from build123d import *

# Parameters (mm, degrees)
SKETCH_1_R          = 2.05
EXTRUDE_1_DEPTH     = 20
FILLET_1_R          = 12
FILLET_2_R          = 8
FILLET_3_R          = 1
FILLET_4_R          = 25
SKETCH_6_R          = 4
CUT_EXTRUDE_5_DEPTH = 3
SKETCH_7_R          = 1.25
CUT_EXTRUDE1_DEPTH  = 10
CUT_EXTRUDE2_START  = -3
SKETCH1_R           = 4
CUT_EXTRUDE2_DEPTH  = 3


with BuildPart() as part:
    # 草图1 → 凸台-拉伸1 (new body)
    with BuildSketch(Plane.XY):
        with BuildLine():
            Line((13.750969278, -0.819876155), (13.750969278, -0.183047918))
            ThreePointArc((13.750969278, -0.183047918), (0.091525986, 13.751882984), (-13.752187557, 0))
            ThreePointArc((-13.752187557, 0), (-24.470803545, -4.924054358), (-35.721657685, -8.467120986))
            ThreePointArc((-35.721657685, -8.467120986), (-46.713142569, -1.298230159), (-54.919247866, -11.538619386))
            Line((-54.919247866, -11.538619386), (-55, -11.852756493))
            Line((-55, -11.852756493), (-55, -22.177115611))
            Line((-55, -22.177115611), (-45.17004572, -22.177115611))
            ThreePointArc((-45.17004572, -22.177115611), (2.155746263, -16.550210115), (49.481538246, -22.177115611))
            Line((49.481538246, -22.177115611), (60, -22.177115611))
            Line((60, -22.177115611), (60, -15.54238751))
            ThreePointArc((60, -15.54238751), (36.185940998, -10.347251745), (13.750969278, -0.819876155))
        make_face()
        with Locations((-45.17004572, -10.942949795)):
            Circle(SKETCH_1_R, mode=Mode.SUBTRACT)
        with BuildLine():
            Line((-7.5, -2.5), (-7.5, 2.5))
            Line((-7.5, 2.5), (-4.330127019, 2.5))
            ThreePointArc((-4.330127019, 2.5), (0, 5), (4.330127019, 2.5))
            Line((4.330127019, 2.5), (7.5, 2.5))
            Line((7.5, 2.5), (7.5, -2.5))
            Line((7.5, -2.5), (4.330127019, -2.5))
            ThreePointArc((4.330127019, -2.5), (0, -5), (-4.330127019, -2.5))
            Line((-4.330127019, -2.5), (-7.5, -2.5))
        make_face(mode=Mode.SUBTRACT)
    extrude(amount=EXTRUDE_1_DEPTH)

    # 圆角1
    fillet_1_edges = [part.edges().sort_by_distance(p)[0] for p in [
        (-13.752187557, 0, 10),
    ]]
    fillet(fillet_1_edges, radius=FILLET_1_R)

    # 圆角2
    fillet_2_edges = [part.edges().sort_by_distance(p)[0] for p in [
        (-35.721657685, -8.467120986, 10),
    ]]
    fillet(fillet_2_edges, radius=FILLET_2_R)

    # 圆角3
    fillet_3_edges = [part.edges().sort_by_distance(p)[0] for p in [
        (60, -15.54238751, 10),
        (60, -22.177115611, 10),
        (-55, -22.177115611, 10),
    ]]
    fillet(fillet_3_edges, radius=FILLET_3_R)

    # 圆角4
    fillet_4_edges = [part.edges().sort_by_distance(p)[0] for p in [
        (13.750969278, -0.819876155, 10),
    ]]
    fillet(fillet_4_edges, radius=FILLET_4_R)

    # 草图6 → 切除-拉伸5 (cut)
    with BuildSketch(Plane(origin=(0, 0, 0), x_dir=(-1, 0, 0), z_dir=(0, 0, -1))):
        with Locations((45.17004572, -10.942949795)):
            Circle(SKETCH_6_R)
    extrude(amount=-CUT_EXTRUDE_5_DEPTH, mode=Mode.SUBTRACT)

    # 草图7 → Cut-Extrude1 (cut)
    with BuildSketch(Plane.XY):
        with Locations((-49.334528207, -19.024990649)):
            Circle(SKETCH_7_R)
        with Locations((54.787690727, -19.024990649)):
            Circle(SKETCH_7_R)
        with Locations((34.734293207, -16.420229149)):
            Circle(SKETCH_7_R)
        with Locations((-28.075836585, -16.420229149)):
            Circle(SKETCH_7_R)
    extrude(amount=CUT_EXTRUDE1_DEPTH, mode=Mode.SUBTRACT)

    # Sketch1 → Cut-Extrude2 (cut)
    with BuildSketch(Plane.XY.offset(20).offset(CUT_EXTRUDE2_START)):
        with Locations(Location((-45.17004572, -10.942949795, 0), (0, 0, 180))):
            Circle(SKETCH1_R)
    extrude(amount=CUT_EXTRUDE2_DEPTH, mode=Mode.SUBTRACT)


solid = part.part
The model under review builds one solid part; all positions refer to its coordinate system, in mm. A direction names the side the tool comes from. Give positions to 0.01 mm unless a question says otherwise; leave off trailing zeros. Loops run counter-clockwise (first coordinate to the right, second up) from the corner with the lowest first, then second, coordinate; pieces in that order, holes last. Notation, with made-up numbers: (62, 34) -> (102, 34) arc R18 ccw to (102, 52) -> close; hole circle Ø5 at (88.5, 31). An arc over 180 degrees is marked (long way). Write each question's results on one line, items separated by ' | '.
1) Draft analysis for pull direction X (two halves, no side actions). For faces 5 (the face through (2, -8, 0)), 6 (the face through (-41.174, -11.119, 18.479)), 7 (the face through (42.14, -12.09, 9.86)), state which applies: pulls with the +X half, pulls with the -X half, needs draft (parallel to the pull), parting line crosses it, or undercut.
Conclusion:
face 5: needs draft | face 6: undercut | face 7: pulls with the +X half
2) Take a section at B-B, the plane z = 7.5. Count the separate pieces of the cut face and the enclosed holes in it, plus the area to 3 significant figures.
Conclusion:
separate pieces: 1 | enclosed holes: 6 | area: 1,760 mm^2
3) Insertion check: pin 1 Ø4 at (y, z) = (-1, 15) entering from -X; pin 2 Ø1 at (x, z) = (-5.5, 5.5) entering from -Y; pin 3 Ø4 at (y, z) = (0.5, 6.5) entering from +X. Each pin has a flat end and moves straight along its axis. Give the tip position at first contact, or say it passes through.
Conclusion:
pin 1: stops at x = -50.85 | pin 2: stops at y = -16.72 | pin 3: stops at x = 17.84
4) Take a section at C-C, the plane y = 7.5. Give the boundary of the cut face in (x, z), plus the area to 3 significant figures.
Conclusion:
outline: (-11.53, 0) -> (11.53, 0) -> (11.53, 20) -> (-11.53, 20) -> close | area: 461 mm^2
5) For line 1 along X through (y, z) = (2, 11); line 2 along Z through (x, y) = (-46.5, -14); line 3 along Y through (x, z) = (3, 12), list the stretches that pass through material, from the lowest coordinate up. Write a range as from..to.
Conclusion:
line 1: x = -14.11..-7.5, 7.5..14.75 | line 2: z = 3..17 | line 3: y = -16.55..-4, 4..13.42
6) Tool access review of faces 1 (the face through (-50, -22.177, 10)), 2 (the face through (6, -2.5, 10)), 3 (the face through (-24.37, -4.885, 9.86)), 4 (the face through (-28.35, -17.64, 4.93)): name each direction out of +Z, -Z, +X, -X, +Y, -Y from which nothing blocks a thin tool from reaching the whole face with its end or side.
Conclusion:
face 1: +Z, -Z, +X, -X, -Y | face 2: +Z, -Z | face 3: +Z, -Z, +Y | face 4: -Z
7) Take a section at A-A, the plane x = -6. Give the boundary of the cut face in (y, z).
Conclusion:
outline: (-16.72, 0) -> (-2.5, 0) -> (-2.5, 20) -> (-16.72, 20) -> close; (2.5, 0) -> (12.37, 0) -> (12.37, 20) -> (2.5, 20) -> close
